For this review, use the dimensioned drawing (mm, ordinates from the lowest corner) and the shaded views. A direction names the side the tool comes from. Give positions to 0.01 mm unless a question says otherwise; leave off trailing zeros. Loops run counter-clockwise (first coordinate to the right, second up) from the corner with the lowest first, then second, coordinate; pieces in that order, holes last. Notation, with made-up numbers: M 72.25,7.25 L 128.25,7.25 A22 cw 128.25,46.25 Z; hole C 21,-19 d2. An arc over 180 degrees is marked long. Use a Markdown table: item, result. Add a question column.
(1) Add section D-D, the plane y = 10.75. Give the boundary of the cut face in (x, z).
(2) Add section A-A, the plane y = 4.5. Give the boundary of the cut face in (x, z).
(3) For probe 1 along Y at (x, z) = (6.5, 2.75); probe 2 along X at (y, z) = (9.25, 1.45); probe 3 along Y at (x, z) = (3.5, 1.85), list the stretches that pass through material, from the lowest coordinate up.
(4) Insertion check: pin 1 Ø1.2 at (x, y) = (3, 10.5) entering from -Z; pin 2 Ø1.5 at (y, z) = (4, 3) entering from -X; pin 3 Ø1.2 at (y, z) = (10, 2) entering from -X; pin 4 Ø1 at (y, z) = (1, 1.5) entering from -X. Each pin has a flat end and moves straight along its axis. Give the tip position at first contact, or say it passes through.
(5) For the marked faces 1, 2, 3, 4 and 5, list the 3-axis set-ups (+Z, -Z, +X, -X, +Y, -Y) from which the entire face can be reached by the end or side of a thin tool; tool diameter is ignored.
(6) Add section C-C, the plane z = 1.1. Give the boundary of the cut face in (x, y).
(7) Add section B-B, the plane x = 3.5. Give the boundary of the cut face in (y, z), then the cut area to 3 significant figures.
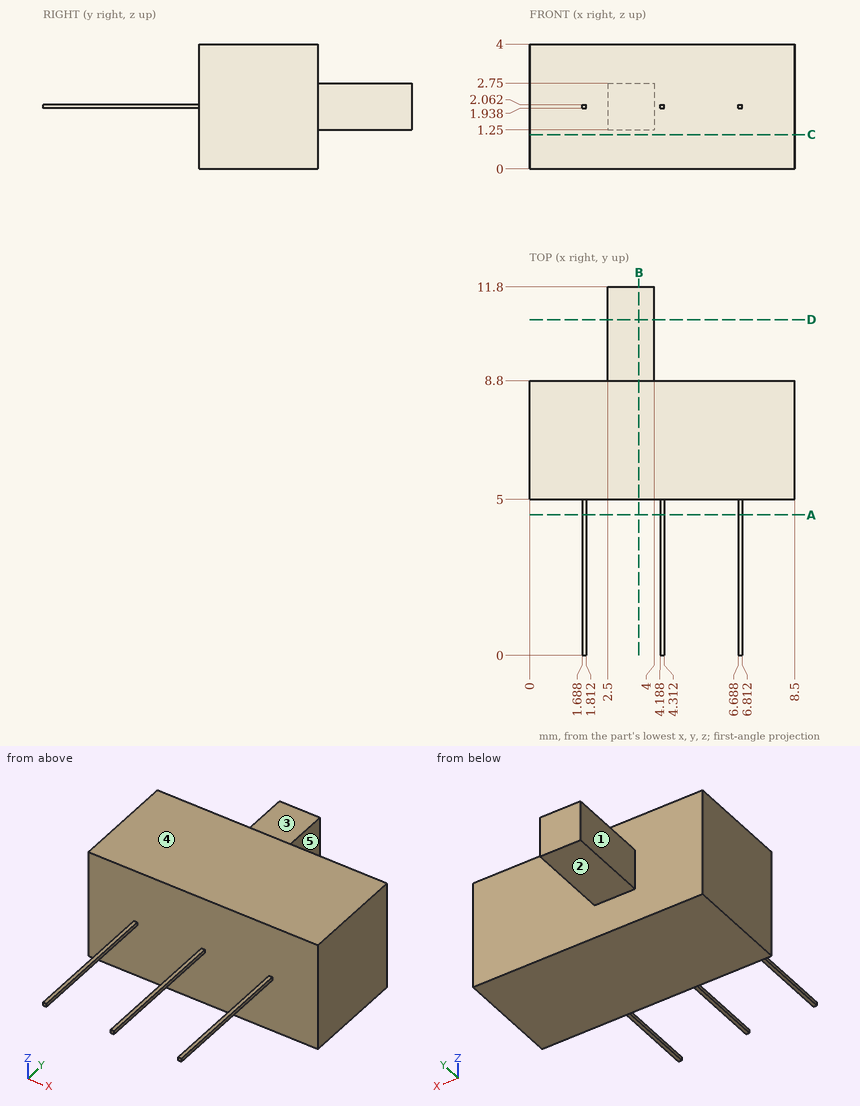
Established:
| question | item | result |
|---|---|---|
| 1 | outline | M 2.5,1.25 L 4,1.25 L 4,2.75 L 2.5,2.75 Z |
| 2 | outline | M 1.69,1.94 L 1.81,1.94 L 1.81,2.06 L 1.69,2.06 Z; M 4.19,1.94 L 4.31,1.94 L 4.31,2.06 L 4.19,2.06 Z; M 6.69,1.94 L 6.81,1.94 L 6.81,2.06 L 6.69,2.06 Z |
| 3 | probe 1 | 5 to 8.8 |
| 3 | probe 2 | 2.5 to 4 |
| 3 | probe 3 | 5 to 11.8 |
| 4 | pin 1 | z = 1.25 |
| 4 | pin 2 | through |
| 4 | pin 3 | x = 2.5 |
| 4 | pin 4 | x = 1.69 |
| 5 | face 1 | +Z, -Z, -X, +Y |
| 5 | face 2 | -Z, +X, -X, +Y |
| 5 | face 3 | +Z, +X, -X, +Y |
| 5 | face 4 | +Z, +X, -X, +Y, -Y |
| 5 | face 5 | +Z, -Z, +X, +Y |
| 6 | outline | M 0,5 L 8.5,5 L 8.5,8.8 L 0,8.8 Z |
| 7 | outline | M 5,0 L 8.8,0 L 8.8,1.25 L 11.8,1.25 L 11.8,2.75 L 8.8,2.75 L 8.8,4 L 5,4 Z |
| 7 | area | 19.7 mm^2 |
